Geometry: see drawing. Coordinates: mm, zero at the bounding-box minimum. Give positions to 0.01 mm unless a question says otherwise; leave off trailing zeros. Loops run counter-clockwise (first coordinate to the right, second up) from the corner with the lowest first, then second, coordinate; pieces in that order, holes last. Notation, with made-up numbers: (34.5, 42) - (76.5, 42) arc R28 ccw to (76.5, 63) - close; hole circle Ø7 at (73, 30.5). An arc over 180 degrees is marked (long way). Use one line per item in the form item = value.
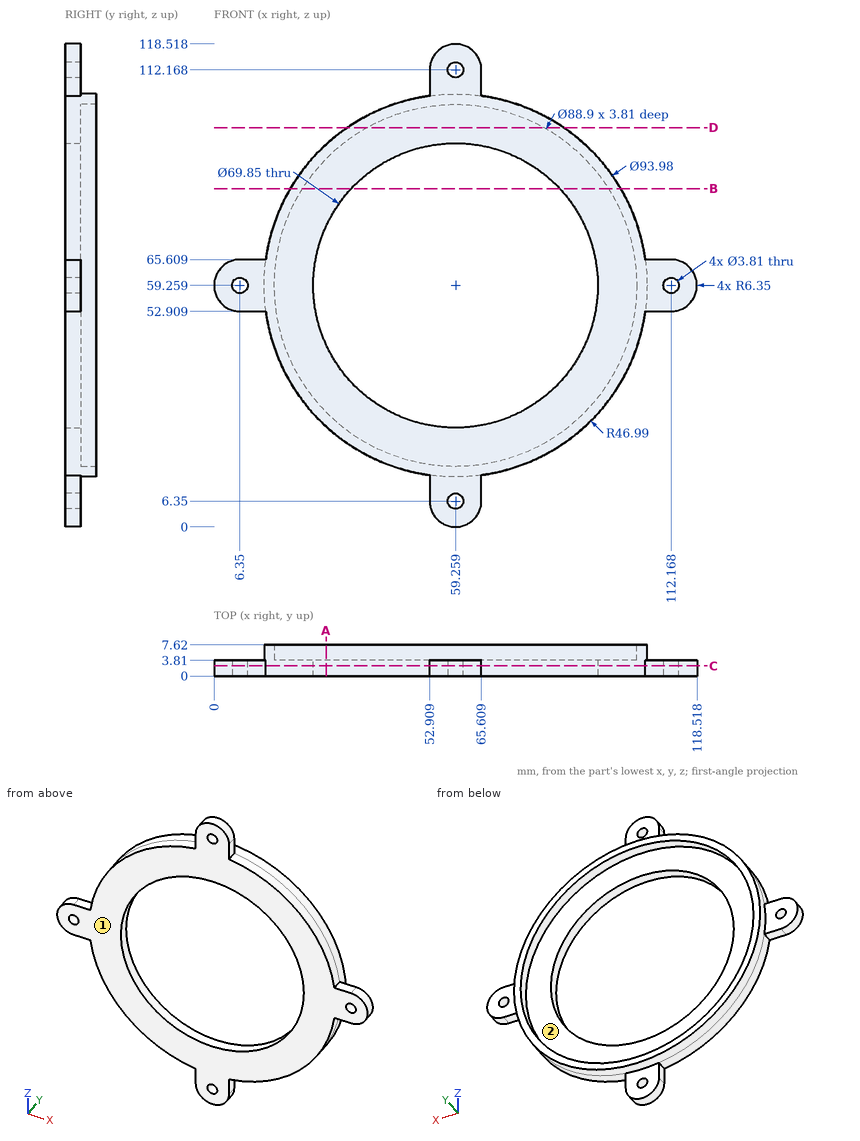
(1) Material intervals for L1, parallel to X at y = 6.5, z = 77 (1 decimal); L2, parallel to X at y = 6, z = 96.5 (1 decimal); L3, parallel to Y at x = 87.5, z = 86, sorted ascending. Write a range as from..to.
Solution:
L1 = 15.7..18.5, 100..102.8
L2 = 30.6..35, 83.5..87.9
L3 = 0..3.81
(2) Cut plane A-A (x = 27.5). Return the cut outline in (y, z).
Solution:
outline = (0, 24.63) - (7.62, 24.63) - (7.62, 28.16) - (3.81, 28.16) - (3.81, 44.73) - (0, 44.73) - close; (0, 73.79) - (3.81, 73.79) - (3.81, 90.36) - (7.62, 90.36) - (7.62, 93.89) - (0, 93.89) - close
(3) Pin query (flat end, axial travel): P1, Ø1.5, axis at x = 32.5, y = 4.5, coming from the -Z side; P2, Ø4, axis at x = 110.5, z = 62, coming from the +Y side; P3, Ø1.9, axis at y = 1.5, z = 9.5, coming from the +X side; P4, Ø5, axis at x = 59.26, z = 112.17, coming from the -Y side. Return the tip coordinate at first contact, or that it passes through.
Solution:
P1 = 20.12
P2 = 3.81
P3 = 65.61
P4 = 0
(4) Cut plane B-B (z = 83). Return the cut outline in (x, y), plus the area to 3 significant figures.
Solution:
outline = (18.71, 0) - (33.64, 0) - (33.64, 3.81) - (21.68, 3.81) - (21.68, 7.62) - (18.71, 7.62) - close; (84.87, 0) - (99.81, 0) - (99.81, 7.62) - (96.84, 7.62) - (96.84, 3.81) - (84.87, 3.81) - close
area = 136 mm2
(5) Cut plane C-C (y = 2.5). Return the cut outline in (x, z) (3 decimals), plus the area to 3 significant figures.
Solution:
outline = (6.35, 52.909) - (12.7, 52.909) arc R46.99 ccw to (52.909, 12.7) - (52.909, 6.35) arc R6.35 ccw to (65.609, 6.35) - (65.609, 12.7) arc R46.99 ccw to (105.818, 52.909) - (112.168, 52.909) arc R6.35 ccw to (112.168, 65.609) - (105.818, 65.609) arc R46.99 ccw to (65.609, 105.818) - (65.609, 112.168) arc R6.35 ccw to (52.909, 112.168) - (52.909, 105.818) arc R46.99 ccw to (12.7, 65.609) - (6.35, 65.609) arc R6.35 ccw to start; hole circle Ø3.81 at (6.35, 59.259); hole circle Ø69.85 at (59.259, 59.259); hole circle Ø3.81 at (59.259, 6.35); hole circle Ø3.81 at (59.259, 112.168); hole circle Ø3.81 at (112.168, 59.259)
area = 3,620 mm2
(6) Pull-direction query (X, two-part tool) for the marked faces 1 and 2; classes: released by +X, released by -X, zero draft, split by the parting line, or undercut.
Solution:
face_1 = zero draft
face_2 = undercut
(7) Cut plane D-D (z = 98). Return the cut outline in (x, y), plus the area to 3 significant figures.
Solution:
outline = (32.67, 0) - (85.85, 0) - (85.85, 7.62) - (81.05, 7.62) - (81.05, 3.81) - (37.47, 3.81) - (37.47, 7.62) - (32.67, 7.62) - close
area = 239 mm2
